Here's how the part is built. I have some questions about the finished solid (model axes, mm). Face numbers are marked on the shaded views. Round coordinates to 2 decimals unless told otherwise and drop trailing zeros. Order: outer loops, then holes, each group sorted by start corner. A loop starts at its lowest first (then second) coordinate and runs counter-clockwise, first axis right, second up. Notation, with made-up numbers: (1, 54) -> (33, 54) arc R8 cw to (33, 65) -> close; hole circle Ø1 at (80.5, 73). An arc over 180 degrees is marked (long way). Use a Markdown table: item, result. Add a question column.
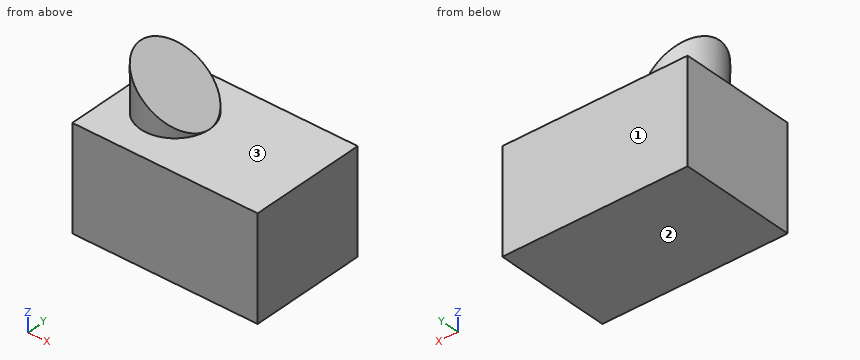
from build123d import *

# Parameters (mm, degrees)
F0_W     = 91.6122980416
F0_H     = 58.0168142915
F1_DEPTH = 50.8
F2_R     = 17.0754278952
F3_DEPTH = 25.4
F4_DEPTH = 50.8
F6_DEPTH = 58.0178142915


with BuildPart() as f1:
    # F0 (on Top) → F1 (new body)
    with BuildSketch(Plane.XY):
        with Locations((-23.8212328404, 42.2187633812)):
            Rectangle(F0_W, F0_H)
    extrude(amount=F1_DEPTH)

    # F2 (on face) → F3 (join)
    with BuildSketch(Plane.XY.offset(50.8)):
        with Locations((-44.6495191595, 43.5129478574)):
            Circle(F2_R)
    extrude(amount=F3_DEPTH)

    # F4 (add): a face of the model
    f4_faces = [f1.faces().sort_by_distance(p)[0] for p in [
        (-19.4842586334, 41.9492815522, 50.8),
    ]]
    extrude(f4_faces, amount=-F4_DEPTH)

    # F5 (on face) → F6 (cut, through all)
    with BuildSketch(Plane.XZ.offset(-13.2103562355)):
        Polygon((-27.5740912643, 76.2), (-61.7249470548, 76.2), (-27.5740912643, 50.8), align=None)
    extrude(amount=-F6_DEPTH, mode=Mode.SUBTRACT)


solid = f1.part
(1) If we mould it in two halves opening along Z, with no side actions, what happens to the marked faces 1, 2 and 3? For each: pulls with the +Z half, pulls with the -Z half, needs draft (parallel to the pull), parting line crosses it, or undercut.
(2) I want a section at C-C on z = 55.5. List the corners of the cut face in (x, y) for me, and give its area (3 significant figures).
(3) I want a section at A-A on y = 39. List the corners of the cut face in (x, z) for me.
(4) I want a section at B-B on x = -57.5. List the corners of the cut face in (y, z) for me, and give its area (3 significant figures).
(5) I want a section at D-D on x = 13. List the corners of the cut face in (y, z) for me.
(6) Please list where these lines run through material, in increasing order: probe 1 along Z at (x, y) = (6, 43); probe 2 along Y at (x, z) = (-56, 67); probe 3 along Y at (x, z) = (-33.5, 52). Write a range as from..to.
(7) I'm going to push flat-ended pins straight in: P1, Ø2, axis at x = -42.5, y = 31.5, coming from the +Z side; P2, Ø6, axis at x = 8.5, y = 46.5, coming from the +Z side; P3, Ø1.5, axis at x = -30.5, y = 48.5, coming from the -Z side; P4, Ø17.5, axis at x = -32.5, y = 28, coming from the +Z side. Where does each tip first touch, or does it pass through?
Output:
| question | item | result |
|---|---|---|
| 1 | face 1 | needs draft |
| 1 | face 2 | pulls with the -Z half |
| 1 | face 3 | pulls with the +Z half |
| 2 | outline | (-33.89, 30.25) -> (-33.89, 56.77) arc R17.08 ccw (long way) to start |
| 2 | area | 799 mm² |
| 3 | outline | (-69.63, 0) -> (21.98, 0) -> (21.98, 50.8) -> (-28.18, 50.8) -> (-28.18, 51.25) -> (-61.12, 75.75) -> (-61.12, 50.8) -> (-69.63, 50.8) -> close |
| 4 | outline | (13.21, 0) -> (71.23, 0) -> (71.23, 50.8) -> (54.76, 50.8) -> (54.76, 73.06) -> (32.27, 73.06) -> (32.27, 50.8) -> (13.21, 50.8) -> close |
| 4 | area | 3,450 mm² |
| 5 | outline | (13.21, 0) -> (71.23, 0) -> (71.23, 50.8) -> (13.21, 50.8) -> close |
| 6 | probe 1 | 0..50.8 |
| 6 | probe 2 | 30.76..56.27 |
| 6 | probe 3 | 30.58..56.45 |
| 7 | P1 | z = 62.65 |
| 7 | P2 | z = 50.8 |
| 7 | P3 | z = 0 |
| 7 | P4 | z = 60.97 |
